Geometry: final body of the model. Coordinates: model frame, mm. Face numbers are marked on the shaded views. A direction names the side the tool comes from. Give positions to 0.01 mm unless a question says otherwise; leave off trailing zeros. Write each loop counter-clockwise with the first axis right and the second up, starting at its lowest first coordinate (ties: lowest second). Pieces come first, ordered by that corner, then holes. Notation, with made-up numbers: (48, 47.5) -> (77, 47.5) arc R15 cw to (77, 69.5) -> close; hole circle Ø7 at (47.25, -12.75). An arc over 180 degrees is marked (long way). Use CSV: the item, a comma, the result in double quotes. Start each with the question number.
1) Section B-B (x = 9.5). Output: boundary loops of the cut face in (y, z).
2) Material intervals for line 1 (X direction, y = 7.5, z = 1.5); line 2 (Y direction, x = 5, z = 0.25); line 3 (X direction, y = 5.75, z = 3.25), sorted ascending. Write a range as [from, to].
3) Section A-A (x = 36). Output: boundary loops of the cut face in (y, z).
4) Set-up query: the marked faces 1, 2 and 3. Return all of +Z, -Z, +X, -X, +Y, -Y with unobstructed straight access to the full face (end or side cutting, diameter ignored); none if empty.
5) Contact query for flat-ended pins moving along their axis: P1, Ø10, axis at x = 24, z = 6, coming from the +Y side; P2, Ø6, axis at x = 22, z = 7, coming from the +Y side; P3, Ø6, axis at x = 39.5, y = 5, coming from the -Z side. Output: stop coordinate, or through.
```python
from build123d import *

# Parameters (mm, degrees)
SKETCH3_R           = 17.357767681
CUT_EXTRUDE1_DEPTH  = 114.5794
SKETCH4_R           = 6.35
BOSS_EXTRUDE1_DEPTH = 12.7
SKETCH5_R           = 8.5344
SKETCH5_R_2         = 6.35
BOSS_EXTRUDE2_DEPTH = 8.89
CUT_EXTRUDE2_START  = -3.81
SKETCH6_R           = 8.5344
SKETCH6_R_2         = 7.2136
CUT_EXTRUDE2_DEPTH  = 2.3622


with BuildPart() as part:
    # Sketch1 → Revolve1 (revolve)
    with BuildSketch(Plane.XY):
        Polygon((12.954, 9.525), (12.954, 8.7376), (13.7414, 8.7376), (13.7414, 9.525), (13.9954, 9.525), (13.9954, 8.7376), (14.7828, 8.7376), (14.7828, 9.525), (15.0368, 9.525), (15.0368, 8.7376), (15.8242, 8.7376), (15.8242, 9.525), (16.0782, 9.525), (16.0782, 8.7376), (16.8656, 8.7376), (16.8656, 9.525), (17.1196, 9.525), (17.1196, 8.7376), (17.907, 8.7376), (17.907, 9.525), (18.161, 9.525), (18.161, 9.271), (19.177, 9.271), (19.177, 8.4836), (19.9644, 8.4836), (19.9644, 9.271), (20.2184, 9.271), (20.2184, 8.4836), (21.0058, 8.4836), (21.0058, 9.271), (21.2598, 9.271), (21.2598, 8.4836), (22.0472, 8.4836), (22.0472, 9.271), (22.3012, 9.271), (22.3012, 8.4836), (23.0886, 8.4836), (23.0886, 9.271), (23.3426, 9.271), (23.3426, 8.4836), (24.13, 8.4836), (24.13, 9.271), (24.384, 9.271), (24.384, 9.017), (25.4, 9.017), (25.4, 8.2296), (26.1874, 8.2296), (26.1874, 9.017), (26.4414, 9.017), (26.4414, 8.2296), (27.2288, 8.2296), (27.2288, 9.017), (27.4828, 9.017), (27.4828, 8.2296), (28.2702, 8.2296), (28.2702, 9.017), (28.5242, 9.017), (28.5242, 8.2296), (29.3116, 8.2296), (29.3116, 9.017), (29.5656, 9.017), (29.5656, 8.2296), (30.353, 8.2296), (30.353, 9.017), (30.607, 9.017), (30.607, 8.763), (31.623, 8.763), (31.623, 7.9756), (32.4104, 7.9756), (32.4104, 8.763), (32.6644, 8.763), (32.6644, 7.9756), (33.4518, 7.9756), (33.4518, 8.763), (33.7058, 8.763), (33.7058, 7.9756), (34.4932, 7.9756), (34.4932, 8.763), (34.7472, 8.763), (34.7472, 7.9756), (35.5346, 7.9756), (35.5346, 8.763), (35.7886, 8.763), (35.7886, 7.9756), (36.576, 7.9756), (36.576, 8.763), (36.83, 8.763), (36.83, 8.509), (37.846, 8.509), (37.846, 7.7216), (38.6334, 7.7216), (38.6334, 8.509), (38.8874, 8.509), (38.8874, 7.7216), (39.6748, 7.7216), (39.6748, 8.509), (39.9288, 8.509), (39.9288, 7.7216), (40.7162, 7.7216), (40.7162, 8.509), (40.9702, 8.509), (40.9702, 7.7216), (41.7576, 7.7216), (41.7576, 8.509), (42.0116, 8.509), (42.0116, 7.7216), (42.799, 7.7216), (42.799, 8.509), (43.053, 8.509), (43.053, 8.255), (44.069, 8.255), (44.069, 7.4676), (44.8564, 7.4676), (44.8564, 8.255), (45.1104, 8.255), (45.1104, 7.4676), (45.8978, 7.4676), (45.8978, 8.255), (46.1518, 8.255), (46.1518, 7.4676), (46.9392, 7.4676), (46.9392, 8.255), (47.1932, 8.255), (47.1932, 7.4676), (47.9806, 7.4676), (47.9806, 8.255), (48.2346, 8.255), (48.2346, 7.4676), (49.022, 7.4676), (49.022, 8.255), (49.276, 8.255), (49.276, 5.999988), (74.676, 5.999988), (74.676, 0), (61.976, 0), (0, 0), (0, 5.999988), (12.7, 5.999988), (12.7, 9.525), align=None)
    revolve(axis=Axis((0, 0, 0), (1, 0, 0)))

    # Sketch3 → Cut-Extrude1 (cut)
    with BuildSketch(Plane(origin=(31.623, 0, 0), x_dir=(0, 0, -1), z_dir=(1, 0, 0))):
        Circle(SKETCH3_R)
    extrude(amount=CUT_EXTRUDE1_DEPTH, mode=Mode.SUBTRACT)

    # Sketch4 → Boss-Extrude1 (add)
    with BuildSketch(Plane(origin=(31.623, 0, 0), x_dir=(0, 0, -1), z_dir=(1, 0, 0))):
        Circle(SKETCH4_R)
    extrude(amount=BOSS_EXTRUDE1_DEPTH)

    # Sketch5 → Boss-Extrude2 (add)
    with BuildSketch(Plane(origin=(31.623, 0, 0), x_dir=(0, 0, -1), z_dir=(1, 0, 0))):
        Circle(SKETCH5_R)
        Circle(SKETCH5_R_2, mode=Mode.SUBTRACT)
    extrude(amount=BOSS_EXTRUDE2_DEPTH)

    # Sketch6 → Cut-Extrude2 (cut)
    with BuildSketch(Plane(origin=(40.513, 0, 0), x_dir=(0, 0, -1), z_dir=(1, 0, 0)).offset(CUT_EXTRUDE2_START)):
        Circle(SKETCH6_R)
        Circle(SKETCH6_R_2, mode=Mode.SUBTRACT)
    extrude(amount=-CUT_EXTRUDE2_DEPTH, mode=Mode.SUBTRACT)


solid = part.part
```
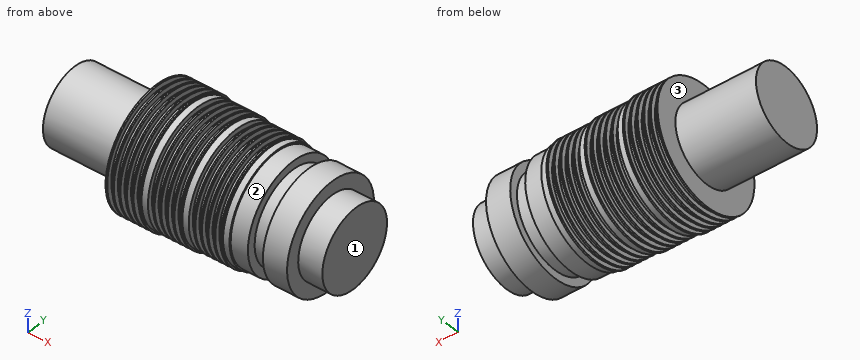
Answers follow:
1,outline,"circle Ø12 at (0, 0)"
2,line 1,"x = [12.7, 34.34], [36.7, 40.51]"
2,line 2,"y = [-5.99, 5.99]"
2,line 3,"x = [12.7, 40.51]"
3,outline,"circle Ø14.43 at (0, 0)"
4,face 1,"+Z, -Z, +X, +Y, -Y"
4,face 2,"+X"
4,face 3,"-X"
5,P1,"stops at y = 9.22"
5,P2,"stops at y = 8.36"
5,P3,"stops at z = -8.3"
